Here's how the part is built. I have some questions about the finished solid (model axes, mm). Face numbers are marked on the shaded views. A direction names the side the tool comes from. Coordinates: 2 decimals unless noted, no trailing zeros. Loops run counter-clockwise (first coordinate to the right, second up) from the corner with the lowest first, then second, coordinate; pieces in that order, holes last. Notation, with made-up numbers: (0, 82.5) -> (55, 82.5) arc R18 cw to (55, 88.5) -> close; hole circle Ø3 at (80, 15.5). An arc over 180 degrees is marked (long way). Answer as a JSON object with one key per item and string values. Group by question number.
1) I want a section at A-A (y = 0). Write out the boundary of the cut face in (x, z), then the cut area to 3 significant figures.
2) If we mould it in two halves opening along Y, with no side actions, what happens to the marked faces 3, 4 and 5? For each: +Y half, -Y half, draft (parallel to the pull), parting line (faces both ways), or undercut.
3) Which directions (+Z, -Z, +X, -X, +Y, -Y) give clear straight access to the entire face, cutting with the end or side of a thin tool? Please do the marked faces 1 and 2.
4) I need wall thicknesses on probe 1 along Y at (x, z) = (3, 0); probe 2 along X at (y, z) = (-0.25, 1.55). Which ranges of each line are inside material? Lowest first, please. Write a range as [from, to].
5) I'm going to push a flat-ended pin straight in: pin 1 (0.7 mm diameter, centred on y = 0, z = 0, fed in from +X). Where does the tip first touch, or does it pass through?
6) I want a section at B-B (x = 4.5). Write out the boundary of the cut face in (y, z).
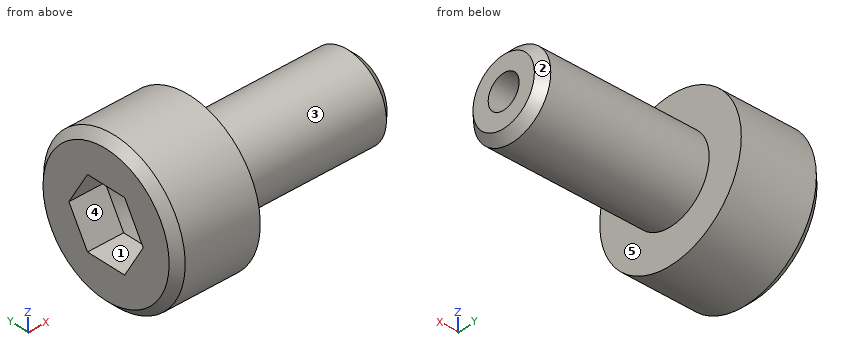
Solid Edge part; units mm, degrees
sketch "Sketch1" plane through (0, 0, 0) normal (0, 0, 1) x (1, 0, 0)
  line L0 (-3, 0) -> (-3, 2.45)
  line L1 (-3, 2.45) -> (-2.7, 2.75)
  line L2 (-2.7, 2.75) -> (0, 2.75)
  line L3 (0, 2.75) -> (0, 1.5)
  line L4 (0, 1.5) -> (5.6935, 1.5)
  line L5 (5.6935, 1.5) -> (6, 1.1935)
  line L6 (6, 1.1935) -> (6, 0)
  line L7 (6, 0) -> (-3, 0)
revolve "RevolvedProtrusion1" add sketch "Sketch1" angle 360 about axis through (6, 0, 0) along (-1, 0, 0)
cosmetic_thread "Thread1"
sketch "Sketch2" plane through (-3, 0, 0) normal (1, 0, 0) x (0, 1, 0)
  line L0 (-0.7217, 1.25) -> (-1.4434, 0)
  line L1 (-1.4434, 0) -> (-0.7217, -1.25)
  line L2 (-0.7217, -1.25) -> (0.7217, -1.25)
  line L3 (0.7217, -1.25) -> (1.4434, 0)
  line L4 (1.4434, 0) -> (0.7217, 1.25)
  line L5 (0.7217, 1.25) -> (-0.7217, 1.25)
extrude "ExtrudedCutout_1" cut sketch "Sketch2" along normal blind 1.3
hole "Hole_1" at (-1.7, 0, 0) direction (1, 0, 0) diameter 1.2 depth 7.7 countersink diameter 2.8868 countersink angle 120
properties part number "SVSS-M3-6-MOS"
Determined:
{
 "1": {"outline": "(-3, -2.45) -> (-2.7, -2.75) -> (0, -2.75) -> (0, -1.5) -> (5.69, -1.5) -> (6, -1.19) -> (6, -0.6) -> (-1.21, -0.6) -> (-1.7, -1.44) -> (-1.7, -1.25) -> (-3, -1.25) -> close; (-3, 1.25) -> (-1.7, 1.25) -> (-1.7, 1.44) -> (-1.21, 0.6) -> (6, 0.6) -> (6, 1.19) -> (5.69, 1.5) -> (0, 1.5) -> (0, 2.75) -> (-2.7, 2.75) -> (-3, 2.45) -> close", "area": "21.4 mm^2"},
 "2": {"face 3": "parting line", "face 4": "undercut", "face 5": "draft"},
 "3": {"face 1": "-X", "face 2": "+X"},
 "4": {"probe 1": "[-1.5, -0.6], [0.6, 1.5]", "probe 2": "[-3, 0]"},
 "5": {"pin 1": "through"},
 "6": {"outline": "circle Ø3 at (0, 0); hole circle Ø1.2 at (0, 0)"}
}
